Geometry: final body of the model. Coordinates: model frame, mm. Face numbers are marked on the shaded views. Give positions to 0.01 mm unless a question says otherwise; leave off trailing zeros. Loops run counter-clockwise (first coordinate to the right, second up) from the corner with the lowest first, then second, coordinate; pieces in that order, holes last.
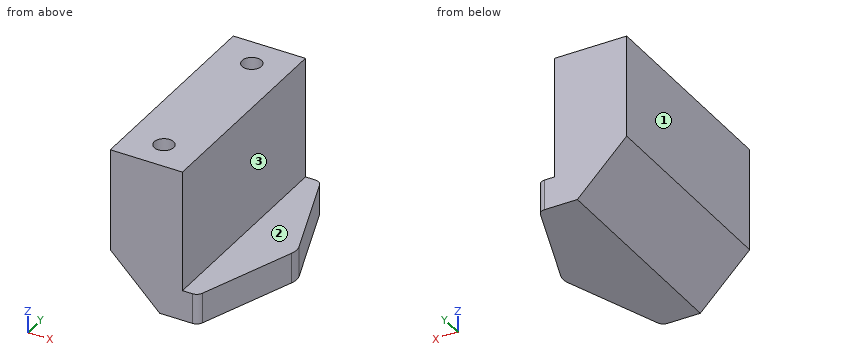
Autodesk Inventor part; units mm, degrees
ref_plane "YZ Plane" through (0, 0, 0) normal (1, 0, 0) x (0, 1, 0)
ref_plane "XZ Plane" through (0, 0, 0) normal (0, 1, 0) x (-1, 0, 0)
ref_plane "XY Plane" through (0, 0, 0) normal (0, 0, 1) x (1, 0, 0)
sketch "Sketch1" plane through (0, 0, 0) normal (0, 0, 1) x (1, 0, 0)
  line L0 (6.0325, -17.78) -> (-6.0325, -17.78)
  line L1 (-6.0325, -17.78) -> (-6.0325, 17.78)
  line L2 (-6.0325, 17.78) -> (6.0325, 17.78)
  line L3 (6.0325, 17.78) -> (6.0325, -17.78)
  line L4 (6.0325, -17.78) -> (-6.0325, 17.78) construction
  line L5 (-6.0325, -17.78) -> (6.0325, 17.78) construction
  point P0 (0, 0)
  dimension "d0" = 12.065
  dimension "d1" = 35.56
extrude "Extrusion1" add sketch "Sketch1" along normal blind 25.4
sketch "Sketch3" plane through (0, 0, 25.4) normal (0, 0, 1) x (1, 0, 0)
  line L0 (6.0325, -17.78) -> (6.0325, 17.78)
  line L1 (0, 26.67) -> (0, -26.67)
  line L2 (-8.4455, 0) -> (8.4455, 0)
  point P0 (0, 12.7)
  point P1 (0, -12.7)
  dimension "d45" = 12.7
  dimension "d46" = 12.7
  dimension "d47" = 0
hole "Hole5" at (0, 12.7, 25.4) at (0, -12.7, 25.4) direction (0, 0, -1) diameter 3.2512 depth 11.811 tip angle 118
sketch "Sketch7" plane through (0, 0, 0) normal (0, 0, -1) x (-1, 0, 0)
  line L0 (-6.0325, -17.78) -> (6.0325, -17.78)
  line L1 (6.0325, 17.78) -> (-6.0325, 17.78)
  line L2 (-6.0325, 17.78) -> (-6.0325, -17.78)
  line L3 (-15.0439, 0) -> (-8.5725, -17.78)
  line L4 (-6.0325, -17.78) -> (-8.5725, -17.78)
  line L5 (-15.0439, 0) -> (-8.5725, 17.78)
  line L6 (-8.5725, 17.78) -> (-6.0325, 17.78)
  line L7 (0, -26.67) -> (0, 26.67)
  line L8 (-19.0666, 0) -> (10.2157, 0)
  point P0 (0, 0)
  dimension "d70" = 70
  dimension "d71" = 70
  dimension "d72" = 2.54
extrude "Extrusion6" add sketch "Sketch7" against normal blind 5.08 contours L4 L3 L8 L2 | L8 L5 L6 L2
fillet "Fillet1" radius 3.175 1 edges at (15.0439, 0, 2.54)
fillet "Fillet2" radius 1.27 2 edges at (8.5725, -17.78, 2.54) (8.5725, 17.78, 2.54)
chamfer "Chamfer1" distance 8.255 angle 45 1 edges at (-6.0325, 0, 0)
properties part number "J005413" material "ALUMINUM, 6061-T651"
Item 1: Section query D-D on x = 11.25. Return loops of the section in (y, z).
Values follow:
outline: (-10.42, 0) - (10.42, 0) - (10.42, 5.08) - (-10.42, 5.08) - close
Item 2: Pin query (flat end, axial travel): pin 1 (5 mm diameter, centred on x = -1, y = 4, fed in from -Z); pin 2 (2 mm diameter, centred on x = 0, y = 12.7, fed in from +Z); pin 3 (2.5 mm diameter, centred on x = 8.5, y = 8, fed in from +Z); pin 4 (1 mm diameter, centred on x = 8.5, z = 8, fed in from -Y). Return the tip coordinate at first contact, or that it passes through.
Values follow:
pin 1: stops at z = 0.72
pin 2: stops at z = 13.21
pin 3: stops at z = 5.08
pin 4: passes through
Item 3: Section query A-A on z = 24. Return loops of the section in (x, y).
Values follow:
outline: (-6.03, -17.78) - (6.03, -17.78) - (6.03, 17.78) - (-6.03, 17.78) - close; hole circle Ø3.25 at (0, -12.7); hole circle Ø3.25 at (0, 12.7)
Item 4: Section query B-B on y = 3.5. Return loops of the section in (x, z) (1 decimal), plus the area to 3 significant figures.
Values follow:
outline: (-6, 8.3) - (2.2, 0) - (13.8, 0) - (13.8, 5.1) - (6, 5.1) - (6, 25.4) - (-6, 25.4) - close
area: 312 mm2
Item 5: Ray query, probe 1 along Y at (x, z) = (0, 17.5); probe 2 along X at (y, z) = (-12.7, 17.25); probe 3 along X at (y, z) = (14, 9.25). Return the intervals inside material, ascending.
Values follow:
probe 1: y = -17.78 to -14.33, -11.07 to 11.07, 14.33 to 17.78
probe 2: x = -6.03 to -1.63, 1.63 to 6.03
probe 3: x = -6.03 to 6.03
Item 6: Draft query along X for the marked faces 1, 2 and 3. Return one class per face: +X half, -X half, draft (parallel to the pull), parting line (faces both ways), or undercut.
Values follow:
face 1: -X half
face 2: draft
face 3: +X half
